Input: part model. Units: mm. Frame: model coordinates. Face numbers are marked on the shaded views. Round coordinates to 2 decimals unless told otherwise and drop trailing zeros. Loops run counter-clockwise (first coordinate to the right, second up) from the corner with the lowest first, then second, coordinate; pieces in that order, holes last. Notation, with made-up numbers: (62.5, -34) -> (91.5, -34) arc R16 ccw to (91.5, -19) -> close; hole circle Ø6 at (-35, 58.25). An arc over 180 degrees is marked (long way). Answer as a JSON object with one key per item and string values. Group by question number.
Item 1: Draft query along X for the marked faces 1, 2 and 3. Return one class per face: released by +X, released by -X, zero draft, split by the parting line, or undercut.
Item 2: Section query C-C on z = 12.5. Return loops of the section in (x, y).
Item 3: Material intervals for line 1 (X direction, y = 2.5, z = 46.5); line 2 (X direction, y = -3.5, z = 12.5); line 3 (Y direction, x = 0, z = 30), sorted ascending. Write a range as [from, to].
Item 4: Section query A-A on y = 0. Return loops of the section in (x, z).
Item 5: Section query D-D on x = 62.5. Return loops of the section in (y, z), and give its area (3 significant figures).
Item 6: Section query B-B on x = 0. Return loops of the section in (y, z), and give its area (3 significant figures).
Item 7: Pin query (flat end, axial travel): pin 1 (20 mm diameter, centred on x = 0, y = 0, fed in from +Z); pin 2 (4 mm diameter, centred on x = 47, z = 23.5, fed in from +Y); pin 3 (6 mm diameter, centred on x = 4.5, z = 12.5, fed in from -Y); pin 4 (12 mm diameter, centred on x = -24.5, z = 39, fed in from +Y). Return the tip coordinate at first contact, or that it passes through.
from build123d import *

# Parameters (mm, degrees)
SKETCH1_R           = 87.5
BOSS_EXTRUDE1_DEPTH = 49
CUT_EXTRUDE1_START  = -15
SKETCH2_R           = 87.5
SKETCH2_R_2         = 86.75
CUT_EXTRUDE1_DEPTH  = 15
M20_TAPPED_HOLE1_D  = 17.5


with BuildPart() as part:
    # Sketch1 → Boss-Extrude1 (new body)
    with BuildSketch(Plane.XY):
        Circle(SKETCH1_R)
    extrude(amount=BOSS_EXTRUDE1_DEPTH)

    # Sketch2 → Cut-Extrude1 (cut)
    with BuildSketch(Plane.XY.offset(49).offset(CUT_EXTRUDE1_START)):
        Circle(SKETCH2_R)
        Circle(SKETCH2_R_2, mode=Mode.SUBTRACT)
    extrude(amount=CUT_EXTRUDE1_DEPTH, mode=Mode.SUBTRACT)

    # M20 Tapped Hole1 (through all)
    with Locations(Plane.XY.offset(49)):
        with Locations((-50, 0), (50, 0)):
            Hole(M20_TAPPED_HOLE1_D / 2)

    # Sketch6 → Ø22.0 (22) Diameter Hole1 (revolve, cut)
    with BuildSketch(Plane(origin=(0, 0, 49), x_dir=(0, -1, 0), z_dir=(1, 0, 0))):
        Polygon((0, 0), (0, 49), (12.5, 49), (11, 47.5), (11, 1.5), (12.5, 0), align=None)
    revolve(axis=Axis((0, 0, 55.35), (0, 0, -1)), mode=Mode.SUBTRACT)


solid = part.part
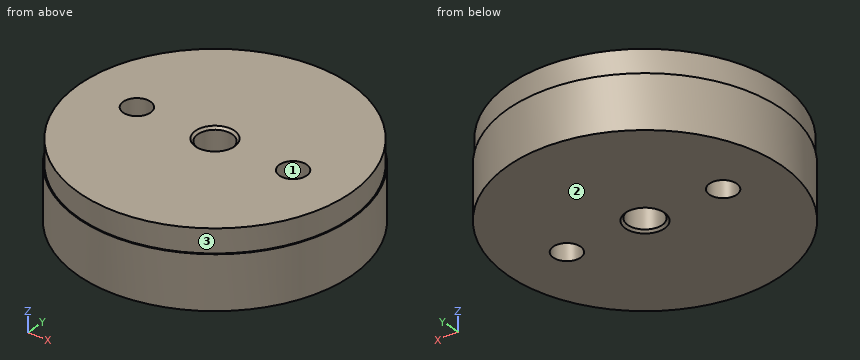
Solved:
{
 "1": {"face 1": "undercut", "face 2": "zero draft", "face 3": "split by the parting line"},
 "2": {"outline": "circle Ø175 at (0, 0); hole circle Ø17.5 at (-50, 0); hole circle Ø22 at (0, 0); hole circle Ø17.5 at (50, 0)"},
 "3": {"line 1": "[-86.71, -58.39], [-41.61, -10.71], [10.71, 41.61], [58.39, 86.71]", "line 2": "[-87.43, -58.02], [-41.98, -10.43], [10.43, 41.98], [58.02, 87.43]", "line 3": "[-87.5, -11], [11, 87.5]"},
 "4": {"outline": "(-87.5, 0) -> (-58.75, 0) -> (-58.75, 49) -> (-86.75, 49) -> (-86.75, 34) -> (-87.5, 34) -> close; (-41.25, 0) -> (-12.5, 0) -> (-11, 1.5) -> (-11, 47.5) -> (-12.5, 49) -> (-41.25, 49) -> close; (11, 1.5) -> (12.5, 0) -> (41.25, 0) -> (41.25, 49) -> (12.5, 49) -> (11, 47.5) -> close; (58.75, 0) -> (87.5, 0) -> (87.5, 34) -> (86.75, 34) -> (86.75, 49) -> (58.75, 49) -> close"},
 "5": {"outline": "(-61.24, 0) -> (61.24, 0) -> (61.24, 34) -> (60.16, 34) -> (60.16, 49) -> (-60.16, 49) -> (-60.16, 34) -> (-61.24, 34) -> close", "area": "5,970 mm²"},
 "6": {"outline": "(-87.5, 0) -> (-12.5, 0) -> (-11, 1.5) -> (-11, 47.5) -> (-12.5, 49) -> (-86.75, 49) -> (-86.75, 34) -> (-87.5, 34) -> close; (11, 1.5) -> (12.5, 0) -> (87.5, 0) -> (87.5, 34) -> (86.75, 34) -> (86.75, 49) -> (12.5, 49) -> (11, 47.5) -> close", "area": "7,470 mm²"},
 "7": {"pin 1": "through", "pin 2": "y = 75.04", "pin 3": "y = -87.49", "pin 4": "y = 84.9"}
}
